Source: CAD feature listing. Evaluate the final solid. Frame: model axes, mm. Round coordinates to 2 decimals unless told otherwise and drop trailing zeros. Loops run counter-clockwise (first coordinate to the right, second up) from the corner with the lowest first, then second, coordinate; pieces in that order, holes last. Notation, with made-up numbers: (0.5, -5) - (21.5, -5) arc R23 cw to (21.5, 3) - close; hole circle Ø8 at (-36, 52). An arc over 180 degrees is marked (long way). One line per question, with ' | ' between items. Start each with the question number.
1. Ray query, line 1 (X direction, y = 135, z = 4.25); line 2 (Y direction, x = -61.5, z = 4.25); line 3 (X direction, y = 167, z = 1). Return the intervals inside material, ascending.
2. Cut plane B-B (z = 2.5). Return loops of the section in (x, y), then the cut area to 3 significant figures.
3. Cut plane C-C (x = -40.5). Return loops of the section in (y, z), then the cut area to 3 significant figures.
4. Cut plane D-D (x = -134). Return loops of the section in (y, z), then the cut area to 3 significant figures.
5. Cut plane A-A (y = 162). Return loops of the section in (x, z).
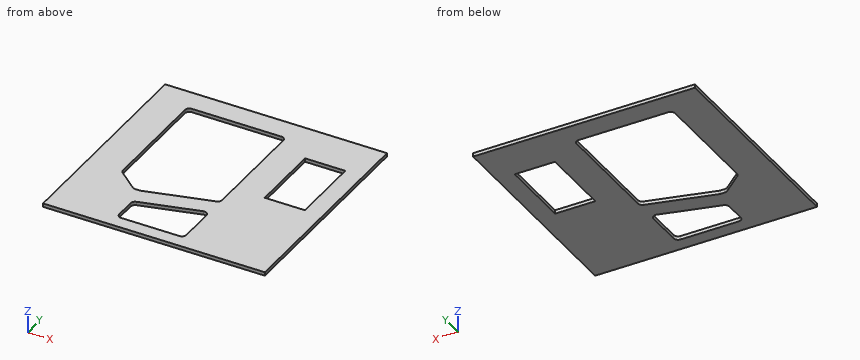
```python
from build123d import *

# Parameters (mm, degrees)
SKETCH1_W           = 496
SKETCH1_H           = 484
BOSS_EXTRUDE1_DEPTH = 8
SKETCH2_W           = 220
SKETCH2_H           = 260
CUT_EXTRUDE1_DEPTH  = 347.600634737
CUT_EXTRUDE2_DEPTH  = 347.600634737
FILLET1_R           = 10
FILLET2_R           = 10
CUT_EXTRUDE3_REACH  = 348.601
SKETCH4_W           = 90
SKETCH4_H           = 160


with BuildPart() as part:
    # Sketch1 → Boss-Extrude1 (new body)
    with BuildSketch(Plane.XY):
        Rectangle(SKETCH1_W, SKETCH1_H)
    extrude(amount=BOSS_EXTRUDE1_DEPTH)

    # Sketch2 → Cut-Extrude1 (cut, through all)
    with BuildSketch(Plane.XY.offset(8)):
        with Locations((-60, 62)):
            Rectangle(SKETCH2_W, SKETCH2_H)
        Polygon((-120.381967555, -109.634472725), (-170, -68), (50, -68), (-105.381967555, -109.634472725), align=None)
    extrude(amount=-CUT_EXTRUDE1_DEPTH, mode=Mode.SUBTRACT)

    # Sketch3 → Cut-Extrude2 (cut, through all)
    with BuildSketch(Plane.XY.offset(8)):
        Polygon((50, -109.411047216), (50, -212), (-100, -212), (-100, -149.603426081), align=None)
    extrude(amount=-CUT_EXTRUDE2_DEPTH, mode=Mode.SUBTRACT)

    # Fillet1
    fillet1_edges = [part.edges().sort_by_distance(p)[0] for p in [
        (50, -212, 4),
        (-100, -212, 4),
        (-100, -149.603426081, 4),
        (50, -109.411047216, 4),
    ]]
    fillet(fillet1_edges, radius=FILLET1_R)

    # Fillet2
    fillet2_edges = [part.edges().sort_by_distance(p)[0] for p in [
        (-170, -68, 4),
        (-170, 192, 4),
        (50, 192, 4),
        (50, -68, 4),
        (-105.381967555, -109.634472725, 4),
        (-120.381967555, -109.634472725, 4),
    ]]
    fillet(fillet2_edges, radius=FILLET2_R)

    # Sketch4 → Cut-Extrude3 (cut, up to next)
    with BuildSketch(Plane.XY.offset(8), mode=Mode.PRIVATE) as cut_extrude3_sk1:
        with Locations((163, 67.567761437)):
            Rectangle(SKETCH4_W, SKETCH4_H)
    cut_extrude3_tool1 = extrude(cut_extrude3_sk1.sketch, amount=-CUT_EXTRUDE3_REACH, mode=Mode.PRIVATE) & part.part
    add(cut_extrude3_tool1.solids().sort_by_distance((163, 67.567761, 8))[0], mode=Mode.SUBTRACT)


solid = part.part
```
Answers follow:
1) line 1: x = -248 to -170, 50 to 118, 208 to 248 | line 2: y = -242 to -212, -139.29 to -97.88, 192 to 242 | line 3: x = -248 to -170, 50 to 248
2) outline: (-248, -242) - (248, -242) - (248, 242) - (-248, 242) - close; hole (-170, -63.34) arc R10 ccw to (-166.43, -71) - (-123.17, -107.29) arc R10 ccw to (-116.74, -109.63) - (-106.7, -109.63) arc R10 ccw to (-104.11, -109.29) - (42.59, -69.99) arc R10 ccw to (50, -60.33) - (50, 182) arc R10 ccw to (40, 192) - (-160, 192) arc R10 ccw to (-170, 182) - close; hole (-100, -202) arc R10 ccw to (-90, -212) - (40, -212) arc R10 ccw to (50, -202) - (50, -122.44) arc R10 ccw to (37.41, -112.78) - (-92.59, -147.62) arc R10 ccw to (-100, -157.28) - close; hole (118, -12.43) - (208, -12.43) - (208, 147.57) - (118, 147.57) - close | area: 151,000 mm2
3) outline: (-242, 0) - (-212, 0) - (-212, 8) - (-242, 8) - close; (-133.66, 0) - (-92.25, 0) - (-92.25, 8) - (-133.66, 8) - close; (192, 0) - (242, 0) - (242, 8) - (192, 8) - close | area: 971 mm2
4) outline: (-242, 0) - (-98.21, 0) - (-98.21, 8) - (-242, 8) - close; (192, 0) - (242, 0) - (242, 8) - (192, 8) - close | area: 1,550 mm2
5) outline: (-248, 0) - (-170, 0) - (-170, 8) - (-248, 8) - close; (50, 0) - (248, 0) - (248, 8) - (50, 8) - close
